Source: CAD feature listing. Evaluate the final solid. Frame: model axes, mm. Face numbers are marked on the shaded views. A direction names the side the tool comes from. Give positions to 0.01 mm unless a question says otherwise; leave off trailing zeros. Order: outer loops, then holes, each group sorted by start corner. A loop starts at its lowest first (then second) coordinate and runs counter-clockwise, first axis right, second up.
```python
from build123d import *

# Parameters (mm, degrees)
F0_W         = 110
F0_H         = 150
F1_DEPTH     = 40
F3_R         = 60
F4_DEPTH     = 50
F6_DEPTH     = 25
F7_W         = 25
F7_H         = 50
F8_DEPTH     = 25
F9_T         = 2.5
F9_T3_DEPTH  = 49.72135955
F9_T5_DEPTH  = 55
F9_T7_DEPTH  = 49.72135955
F9_T10_ANGLE = 118.9875137878
F9_T12_ANGLE = 118.9875137878


# Not quite as in the source:
# - a shell that OpenCascade refuses in one call is made with other operations: the cavity is built on its own and cut out


with BuildPart() as f1:
    # F0 (on Top) → F1 (new body)
    with BuildSketch(Plane.XY):
        Rectangle(F0_W, F0_H)
    extrude(amount=F1_DEPTH)

    # F3 (on offset) → F4 (cut)
    with BuildSketch(Plane.YZ.offset(-47)):
        with Locations((16.3003693058, 70.4579347266)):
            Circle(F3_R)
    extrude(amount=F4_DEPTH, mode=Mode.SUBTRACT)

    # F5 (on face) → F6 (join)
    with BuildSketch(Plane.YZ.offset(55)):
        Polygon((-5, 0), (5, 0), (25, 40), (-25, 40), align=None)
    extrude(amount=F6_DEPTH)

    # F7 (on face) → F8 (join)
    with BuildSketch(Plane.XY.offset(40)):
        with Locations((67.5, 0)):
            Rectangle(F7_W, F7_H)
    extrude(amount=F8_DEPTH)

    # F9: shell of thickness 2.5, made by hand


with BuildPart() as f9_core1:
    # F9_t2: copy of F1
    add(f1.part)

    # the walls: a layer under each face that stays
    f9_faces = [f9_core1.faces().sort_by_distance(p)[0] for p in [
        (0, -75, 20),
        (-55, 0, 20),
        (55, -40, 20),
        (12.5, 0, 0),
        (-36.6666666667, -50, 40),
        (0, 75, 20),
        (67.5, -15, 20),
        (80, 0, 32.5),
        (67.5, 15, 20),
        (55, 40, 20),
        (55, 0, 52.5),
        (3, 16.3003693058, 25.2289673633),
        (-22, 16.3003693058, 10.4579347266),
        (-47, 16.3003693058, 25.2289673633),
        (67.5, -25, 52.5),
        (67.5, 25, 52.5),
    ]]
    thicken(f9_faces, amount=-F9_T, mode=Mode.SUBTRACT)

    # F9_s4 → F9_t3 (cut)
    with BuildSketch(Plane(origin=(0, -22.1180339887, 44.2360679775), x_dir=(1, 0, 0), z_dir=(0, 0.4472135955, -0.894427191))):
        Polygon((55.025, 4.497135955), (52.5, 4.472135955), (52.5, 1.972135955), (55, 1.972135955), align=None)
    extrude(amount=F9_T3_DEPTH, mode=Mode.SUBTRACT)

    # F9_s6 → F9_t5 (cut)
    with BuildSketch(Plane.XZ.offset(-27.5)):
        Polygon((54.975, 40.025), (55, 37.5), (57.5, 37.5), (57.5, 40), align=None)
    extrude(amount=F9_T5_DEPTH, mode=Mode.SUBTRACT)

    # F9_s8 → F9_t7 (cut)
    with BuildSketch(Plane(origin=(0, -0.1180339887, -0.2360679775), x_dir=(1, 0, 0), z_dir=(0, 0.4472135955, 0.894427191))):
        Polygon((55.025, 4.497135955), (55, 1.972135955), (52.5, 1.972135955), (52.5, 4.472135955), align=None)
    extrude(amount=F9_T7_DEPTH, mode=Mode.SUBTRACT)

    # F9_s9 → F9_t10 (revolve, cut)
    with BuildSketch(Plane(origin=(0, -26.6152201498, 45.172421505), x_dir=(1, 0, 0), z_dir=(0, -0.5076322454, 0.8615738525))):
        Polygon((2.975, -10.1643084047), (5.5, -10.1893084047), (5.5, -12.6893084047), (3, -12.6893084047), align=None)
    revolve(axis=Axis((3, 16.3003693058, 70.4579347266), (1, 0, 0)), revolution_arc=F9_T10_ANGLE, mode=Mode.SUBTRACT)

    # F9_s11 → F9_t12 (revolve, cut)
    with BuildSketch(Plane(origin=(0, -26.6152201498, 45.172421505), x_dir=(1, 0, 0), z_dir=(0, -0.5076322454, 0.8615738525))):
        Polygon((-46.975, -10.1643084047), (-47, -12.6893084047), (-49.5, -12.6893084047), (-49.5, -10.1893084047), align=None)
    revolve(axis=Axis((-47, 16.3003693058, 70.4579347266), (1, 0, 0)), revolution_arc=F9_T12_ANGLE, mode=Mode.SUBTRACT)


with BuildPart() as f1_1:
    add(f1.part)

    # what is left inside the walls is the cavity
    f9_cavity = [f9_core1.part.solids().sort_by_distance(p)[0] for p in [
        (12.5, -24.166667, 2.525),
    ]]
    add(f9_cavity, mode=Mode.SUBTRACT)


solid = f1_1.part
```
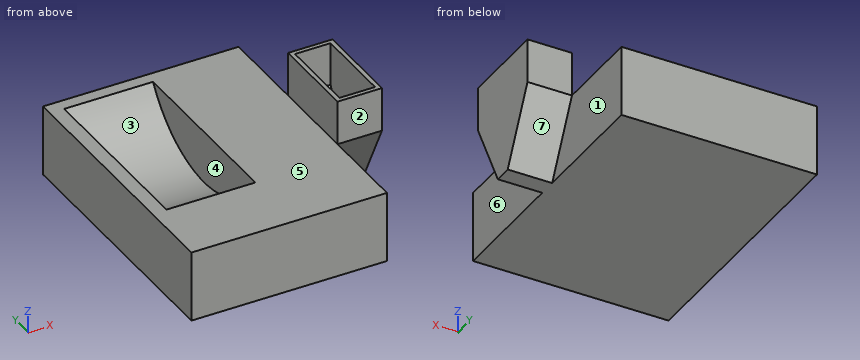
1) Section query B-B, the plane y = -52. Return the cut outline in (x, z), and give its area (3 significant figures).
Report:
outline: (-55, 0) - (55, 0) - (55, 40) - (-55, 40) - close; hole (-52.5, 2.5) - (52.5, 2.5) - (52.5, 37.5) - (-52.5, 37.5) - close
area: 725 mm2
2) Reachability of the marked faces 4, 5, 6 and 7 from +Z, -Z, +X, -X, +Y, -Y: full face, straight path, thin tool, end or side. Return the list, or none.
Report:
face 4: +Z
face 5: +Z, -X, +Y, -Y
face 6: -Z, +X, -Y
face 7: -Z, +X, +Y
3) Pin query (flat end, axial travel): pin 1 (12 mm diameter, centred on x = -11, y = 18.5, fed in from +Z); pin 2 (20 mm diameter, centred on x = 70, z = 58.5, fed in from +Y); pin 3 (6 mm diameter, centred on x = 63.5, z = 52.5, fed in from -Y). Return the tip coordinate at first contact, or that it passes through.
Report:
pin 1: stops at z = 11.02
pin 2: stops at y = 25
pin 3: stops at y = -25
4) Section query D-D, the plane z = 52.5. Return the cut outline in (x, y), and give its area (3 significant figures).
Report:
outline: (55, -25) - (80, -25) - (80, 25) - (55, 25) - close; hole (57.5, -22.5) - (77.5, -22.5) - (77.5, 22.5) - (57.5, 22.5) - close
area: 350 mm2
5) Material intervals for L1, parallel to X at y = 33.5, z = 11.5; L2, parallel to X at y = -6, z = 37; L3, parallel to X at y = 39, z = 19.5, sorted ascending.
Report:
L1: x = -55 to -52.5, -49.5 to 5.5, 52.5 to 55
L2: x = -55 to -52.5, -49.5 to -47, 3 to 5.5, 77.5 to 80
L3: x = -55 to -52.5, -49.5 to -47, 3 to 5.5, 52.5 to 55
6) Section query C-C, the plane x = -10.5. Return the cut outline in (y, z).
Report:
outline: (-75, 0) - (75, 0) - (75, 40) - (67.99, 40) arc R60 cw to (-35.39, 40) - (-75, 40) - close; hole (-72.5, 2.5) - (72.5, 2.5) - (72.5, 37.5) - (69.4, 37.5) arc R62.5 cw to (-36.8, 37.5) - (-72.5, 37.5) - close
7) Draft query along X for the marked faces 1, 2 and 3. Return one class per face: +X half, -X half, draft (parallel to the pull), parting line (faces both ways), or undercut.
Report:
face 1: +X half
face 2: draft
face 3: undercut
8) Section query A-A, the plane z = 20.5. Return the cut outline in (x, y), and give its area (3 significant figures).
Report:
outline: (-55, -75) - (55, -75) - (55, -15.25) - (80, -15.25) - (80, 15.25) - (55, 15.25) - (55, 75) - (-55, 75) - close; (-49.5, -21.26) - (5.5, -21.26) - (5.5, 53.86) - (-49.5, 53.86) - close; hole (-52.5, -72.5) - (52.5, -72.5) - (52.5, -12.45) - (77.5, -12.45) - (77.5, 12.45) - (52.5, 12.45) - (52.5, 72.5) - (-52.5, 72.5) - close; hole (-47, -16.93) - (3, -16.93) - (3, 49.53) - (-47, 49.53) - close
area: 2,220 mm2
